Input: part model. Units: mm. Frame: model coordinates. A direction names the side the tool comes from. Give positions to 0.01 mm unless a question says otherwise; leave off trailing zeros. Order: outer loops, then holes, each group sorted by start corner. A loop starts at its lowest first (then second) coordinate and runs counter-clockwise, first axis right, second up. Notation, with made-up numbers: (22.25, 89) - (75.25, 89) arc R23 ccw to (75.25, 116) - close; hole circle Ø4 at (51, 68.5). An arc over 180 degrees is marked (long way). Use a Markdown table: item, result.
from build123d import *

# Parameters (mm, degrees)
SKETCH_1_R          = 4.5
EXTRUDE_1_DEPTH     = 4.8
SKETCH_2_W          = 11.2
SKETCH_2_H          = 13.8
EXTRUDE_2_DEPTH     = 1.8
FILLET_1_R          = 0.4
SKETCH_4_R          = 2
EXTRUDE_3_DEPTH     = 10
CUT_EXTRUDE_1_DEPTH = 4
SKETCH_7_R          = 1.1
CUT_EXTRUDE_2_DEPTH = 16.7213231


with BuildPart() as part:
    # Эскиз1 → Бобышка-Вытянуть1 (new body)
    with BuildSketch(Plane.XY):
        Circle(SKETCH_1_R)
    extrude(amount=EXTRUDE_1_DEPTH)

    # Эскиз2 → Бобышка-Вытянуть2 (add)
    with BuildSketch(Plane.XY.offset(4.8)):
        with Locations((0.2, 0.5)):
            Rectangle(SKETCH_2_W, SKETCH_2_H)
    extrude(amount=EXTRUDE_2_DEPTH)

    # Скругление1
    fillet_1_edges = [part.edges().sort_by_distance(p)[0] for p in [
        (-4.5, 0, 0),
    ]]
    fillet(fillet_1_edges, radius=FILLET_1_R)

    # Эскиз4 → Бобышка-Вытянуть3 (add)
    with BuildSketch(Plane.XY.offset(6.6)):
        with Locations((-3.35, -1.6)):
            Circle(SKETCH_4_R)
    extrude(amount=EXTRUDE_3_DEPTH)

    # Эскиз3 → Вырез-Вытянуть1 (cut)
    with BuildSketch(Plane(origin=(0, 0, 0), x_dir=(-1, 0, 0), z_dir=(0, 0, -1))):
        Polygon((-3, -1.73), (3, -1.73), (0, 3.466152423), align=None)
    extrude(amount=-CUT_EXTRUDE_1_DEPTH, mode=Mode.SUBTRACT)

    # Эскиз7 → Вырез-Вытянуть2 (cut, through all)
    with BuildSketch(Plane(origin=(0, 0, 4), x_dir=(-1, 0, 0), z_dir=(0, 0, -1))):
        with Locations((0.003552103, 0)):
            Circle(SKETCH_7_R)
    extrude(amount=-CUT_EXTRUDE_2_DEPTH, mode=Mode.SUBTRACT)


solid = part.part
1. Section query B-B (z = 11.5). Return loops of the section in (x, y).
Response:
| item | result |
|---|---|
| outline | circle Ø4 at (-3.35, -1.6) |
2. Mould query, pull axis X, two halves, no side actions, for faces 4 (the face through (0, 7.4, 6)), 5 (the face through (1.48, 0.9, 1.97)), 6 (the face through (-0.59, 4.46, 2.57)). Classes: pulls with the +X half, pulls with the -X half, needs draft (parallel to the pull), parting line crosses it, or undercut.
Response:
| item | result |
|---|---|
| face 4 | needs draft |
| face 5 | undercut |
| face 6 | parting line crosses it |
3. Set-up query: faces 1 (the face through (5.8, 0, 6)), 2 (the face through (0, 5, 4.8)), 3 (the face through (-4.937, -2.817, 11.53)). Return all of +Z, -Z, +X, -X, +Y, -Y with unobstructed straight access to the full face (end or side cutting, diameter ignored); none if empty.
Response:
| item | result |
|---|---|
| face 1 | +Z, -Z, +X, +Y, -Y |
| face 2 | -Z |
| face 3 | +Z |
4. Section query C-C (x = 5.25). Return loops of the section in (y, z), then the cut area to 3 significant figures.
Response:
| item | result |
|---|---|
| outline | (-6.4, 4.8) - (7.4, 4.8) - (7.4, 6.6) - (-6.4, 6.6) - close |
| area | 24.8 mm^2 |
5. Section query A-A (y = 0). Return loops of the section in (x, z).
Response:
| item | result |
|---|---|
| outline | (-5.4, 4.8) - (-4.5, 4.8) - (-4.5, 0.4) arc R0.4 ccw to (-4.1, 0) - (-2, 0) - (-2, 4) - (-1.1, 4) - (-1.1, 6.6) - (-2.15, 6.6) - (-2.15, 16.6) - (-4.55, 16.6) - (-4.55, 6.6) - (-5.4, 6.6) - close; (1.1, 4) - (2, 4) - (2, 0) - (4.1, 0) arc R0.4 ccw to (4.5, 0.4) - (4.5, 4.8) - (5.8, 4.8) - (5.8, 6.6) - (1.1, 6.6) - close |
6. Pin query (flat end, axial travel): pin 1 (2 mm diameter, centred on x = 0.5, y = 0.5, fed in from +Z); pin 2 (5 mm diameter, centred on x = 2.5, z = 15, fed in from -Y); pin 3 (1.2 mm diameter, centred on x = -1, z = 1.5, fed in from +Y); pin 4 (2 mm diameter, centred on x = -4, z = 9.5, fed in from -Y). Return the tip coordinate at first contact, or that it passes through.
Response:
| item | result |
|---|---|
| pin 1 | stops at z = 6.6 |
| pin 2 | passes through |
| pin 3 | stops at y = 4.48 |
| pin 4 | stops at y = -3.6 |
7. Material intervals for line 1 along Z through (x, y) = (2.5, 3); line 2 along Z through (x, y) = (-4, 4.5); line 3 along Y through (x, z) = (-2, 2.75), sorted ascending.
Response:
| item | result |
|---|---|
| line 1 | z = 0 to 6.6 |
| line 2 | z = 4.8 to 6.6 |
| line 3 | y = -4.03 to -1.73, 0 to 4.03 |
